from build123d import *

# Parameters (mm, degrees)
CROQUIS1_R              = 25
SALIENTE_EXTRUIR1_DEPTH = 10
CROQUIS2_R              = 20
SALIENTE_EXTRUIR3_DEPTH = 40
CROQUIS4_W              = 13
CROQUIS4_H              = 23
CORTAR_EXTRUIR2_DEPTH   = 40


with BuildPart() as part:
    # Croquis1 → Saliente-Extruir1 (new body)
    with BuildSketch(Plane(origin=(0, 0, 0), x_dir=(1, 0, 0), z_dir=(0, 1, 0))):
        Circle(CROQUIS1_R)
    extrude(amount=SALIENTE_EXTRUIR1_DEPTH)

    # Croquis2 → Saliente-Extruir3 (add)
    with BuildSketch(Plane(origin=(0, 10, 0), x_dir=(1, 0, 0), z_dir=(0, 1, 0))):
        Circle(CROQUIS2_R)
    extrude(amount=SALIENTE_EXTRUIR3_DEPTH)

    # Croquis4 → Cortar-Extruir2 (cut)
    with BuildSketch(Plane(origin=(0, 0, 0), x_dir=(0, 0, -1), z_dir=(1, 0, 0))):
        with Locations((0, 38.5)):
            Rectangle(CROQUIS4_W, CROQUIS4_H)
    extrude(amount=CORTAR_EXTRUIR2_DEPTH, mode=Mode.SUBTRACT)


solid = part.part
Source: CAD feature listing. Evaluate the final solid. Frame: model axes, mm. A direction names the side the tool comes from. Round coordinates to 2 decimals unless told otherwise and drop trailing zeros. Loops run counter-clockwise (first coordinate to the right, second up) from the corner with the lowest first, then second, coordinate; pieces in that order, holes last. Notation, with made-up numbers: (16, 22) -> (50, 22) arc R9 cw to (50, 37) -> close; hole circle Ø1 at (19.25, 5.25). An arc over 180 degrees is marked (long way). Answer as a JSON object with one key per item and string values. Group by question number.
Q1. Contact query for flat-ended pins moving along their axis: P1, Ø2, axis at y = 30, z = -9.5, coming from the -X side; P2, Ø1, axis at y = 39, z = 1, coming from the +X side; P3, Ø6, axis at y = 27.5, z = -10.5, coming from the -X side. Output: stop coordinate, or through.
Q2. Access query for faces 1 (the flat face through (9, 38, -6.5)), 2 (the flat face through (-1, 50, 0)), 3 (the cylindrical face through (-16, 30, 12)). Directions: +Z, -Z, +X, -X, +Y, -Y. A direction counts if a zero-diameter tool reaches every point of the face in a straight line with its end or side. Return the directions, or none.
Q3. Mould query, pull axis Z, two halves, no side actions, for faces 4 (the flat face through (-11, 10, -17)), 5 (the cylindrical face through (23.846, 4.93, -7.509)), 6 (the flat face through (10, 27, 0)). Classes: pulls with the +Z half, pulls with the -Z half, needs draft (parallel to the pull), parting line crosses it, or undercut.
Q4. Section query D-D (x = -1). Output: boundary loops of the cut face in (y, z), plus the area to 3 significant figures.
Q5. Section query B-B (x = 6). Output: boundary loops of the cut face in (y, z).
Q6. Section query A-A (z = 1). Output: boundary loops of the cut face in (x, y).
Q7. Section query C-C (y = 15). Output: boundary loops of the cut face in (x, z), plus the area to 3 significant figures.
Q8. Ray query, line 1 (X direction, y = 8, z = -15); line 2 (X direction, y = 45.5, z = 0); line 3 (Z direction, x = 11.5, y = 40). Return the intervals inside material, ascending. Write a range as from..to.
Completed:
{
 "1": {"P1": "x = -18.1", "P2": "x = 0", "P3": "x = -18.54"},
 "2": {"face 1": "+X, +Y", "face 2": "+Z, -Z, +X, -X, +Y", "face 3": "+Y"},
 "3": {"face 4": "needs draft", "face 5": "parting line crosses it", "face 6": "undercut"},
 "4": {"outline": "(0, -24.98) -> (10, -24.98) -> (10, -19.97) -> (50, -19.97) -> (50, 19.97) -> (10, 19.97) -> (10, 24.98) -> (0, 24.98) -> close", "area": "2,100 mm²"},
 "5": {"outline": "(0, -24.27) -> (10, -24.27) -> (10, -19.08) -> (50, -19.08) -> (50, -6.5) -> (27, -6.5) -> (27, 6.5) -> (50, 6.5) -> (50, 19.08) -> (10, 19.08) -> (10, 24.27) -> (0, 24.27) -> close"},
 "6": {"outline": "(-24.98, 0) -> (24.98, 0) -> (24.98, 10) -> (19.97, 10) -> (19.97, 27) -> (0, 27) -> (0, 50) -> (-19.97, 50) -> (-19.97, 10) -> (-24.98, 10) -> close"},
 "7": {"outline": "circle Ø40 at (0, 0)", "area": "1,260 mm²"},
 "8": {"line 1": "-20..20", "line 2": "-20..0", "line 3": "-16.36..-6.5, 6.5..16.36"}
}
